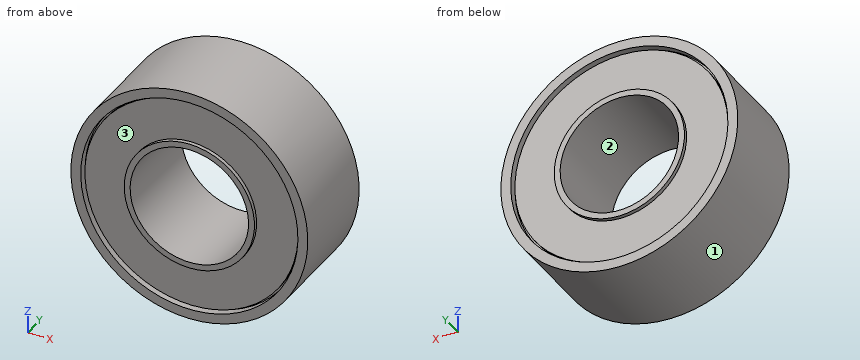
```python
from build123d import *

# Parameters (mm, degrees)
SKETCH_1_R          = 3
SKETCH_1_R_2        = 1.5
EXTRUDE_1_DEPTH     = 2.4
SKETCH_2_R          = 2.75
SKETCH_2_R_2        = 1.65
CUT_EXTRUDE_1_DEPTH = 0.1
CUT_EXTRUDE_START   = -0.1
SKETCH_3_R          = 2.75
SKETCH_3_R_2        = 1.65
CUT_EXTRUDE_2_DEPTH = 0.1
SKETCH_4_R          = 2.75
SKETCH_4_R_2        = 2.7
CUT_EXTRUDE_3_DEPTH = 0.1
SKETCH_5_R          = 2.75
SKETCH_5_R_2        = 2.7
CUT_EXTRUDE_4_DEPTH = 0.1


with BuildPart() as part:
    # 草图1 → 凸台-拉伸1 (new body)
    with BuildSketch(Plane(origin=(0, 0, 0), x_dir=(1, 0, 0), z_dir=(0, 1, 0))):
        with Locations(Location((0, 0, 0), (0, 0, 270))):
            Circle(SKETCH_1_R)
        with Locations(Location((0, 0, 0), (0, 0, 270))):
            Circle(SKETCH_1_R_2, mode=Mode.SUBTRACT)
    extrude(amount=EXTRUDE_1_DEPTH)

    # 草图2 → 切除-拉伸1 (cut)
    with BuildSketch(Plane(origin=(0, 2.4, 0), x_dir=(1, 0, 0), z_dir=(0, 1, 0))):
        with Locations(Location((0, 0, 0), (0, 0, 270))):
            Circle(SKETCH_2_R)
        with Locations(Location((0, 0, 0), (0, 0, 270))):
            Circle(SKETCH_2_R_2, mode=Mode.SUBTRACT)
    extrude(amount=-CUT_EXTRUDE_1_DEPTH, mode=Mode.SUBTRACT)

    # 草图3 → 切除-拉伸2 (cut)
    with BuildSketch(Plane.XZ.offset(CUT_EXTRUDE_START)):
        with Locations(Location((0, 0, 0), (0, 0, 90))):
            Circle(SKETCH_3_R)
        with Locations(Location((0, 0, 0), (0, 0, 90))):
            Circle(SKETCH_3_R_2, mode=Mode.SUBTRACT)
    extrude(amount=CUT_EXTRUDE_2_DEPTH, mode=Mode.SUBTRACT)

    # 草图4 → 切除-拉伸3 (cut)
    with BuildSketch(Plane.XZ.offset(-0.1).offset(CUT_EXTRUDE_START)):
        with Locations(Location((0, 0, 0), (0, 0, 90))):
            Circle(SKETCH_4_R)
        with Locations(Location((0, 0, 0), (0, 0, 270))):
            Circle(SKETCH_4_R_2, mode=Mode.SUBTRACT)
    extrude(amount=CUT_EXTRUDE_3_DEPTH, mode=Mode.SUBTRACT)

    # 草图5 → 切除-拉伸4 (cut)
    with BuildSketch(Plane(origin=(0, 2.3, 0), x_dir=(1, 0, 0), z_dir=(0, 1, 0))):
        with Locations(Location((0, 0, 0), (0, 0, 270))):
            Circle(SKETCH_5_R)
        with Locations(Location((0, 0, 0), (0, 0, 90))):
            Circle(SKETCH_5_R_2, mode=Mode.SUBTRACT)
    extrude(amount=-CUT_EXTRUDE_4_DEPTH, mode=Mode.SUBTRACT)


solid = part.part
```
Check sheet for the modelled part. Datum: model origin and axes. Units: mm. Face numbers are marked on the shaded views. Round coordinates to 2 decimals unless told otherwise and drop trailing zeros. Order: outer loops, then holes, each group sorted by start corner. A loop starts at its lowest first (then second) coordinate and runs counter-clockwise, first axis right, second up.
1) Mould release check, pull along X, two halves, no side actions. Record for the marked faces 1, 2 and 3: +X half, -X half, draft (parallel to the pull), parting line (faces both ways), or undercut.
2) Section check C-C (y = 0.5). Record the boundary of the cut face in (x, z).
3) Scan lines: line 1 (X direction, y = 0.45, z = 0); line 2 (X direction, y = 0.7, z = 1.05); line 3 (Y direction, x = -1.1, z = -2.15). Record each from-to range of solid material in increasing order.
4) Go/stop test with a flat-tipped pin: pin 1 Ø1.6 at (x, z) = (0, -0.5) entering from -Y. Record where the tip stops, or that it passes through.
5) Section check D-D (x = 2.1). Record the boundary of the cut face in (y, z).
Result:
1. face 1: parting line
1. face 2: undercut
1. face 3: undercut
2. outline: circle Ø6 at (0, 0); hole circle Ø3 at (0, 0)
3. line 1: x = -3 to -1.5, 1.5 to 3
3. line 2: x = -2.81 to -1.07, 1.07 to 2.81
3. line 3: y = 0.1 to 2.3
4. pin 1: passes through
5. outline: (0, -2.14) - (2.4, -2.14) - (2.4, -1.78) - (2.2, -1.78) - (2.2, -1.7) - (2.3, -1.7) - (2.3, 1.7) - (2.2, 1.7) - (2.2, 1.78) - (2.4, 1.78) - (2.4, 2.14) - (0, 2.14) - (0, 1.78) - (0.2, 1.78) - (0.2, 1.7) - (0.1, 1.7) - (0.1, -1.7) - (0.2, -1.7) - (0.2, -1.78) - (0, -1.78) - close
